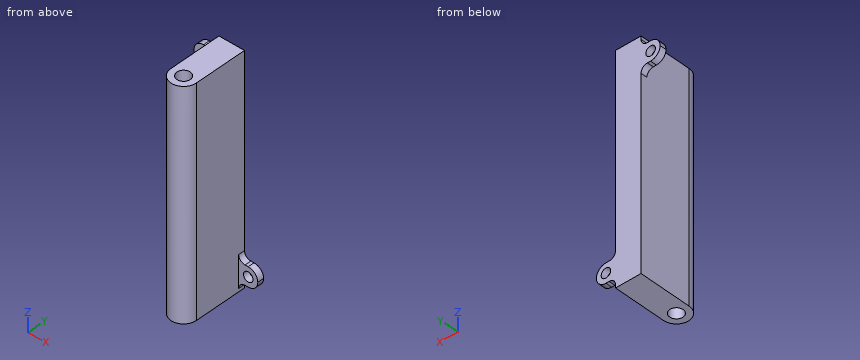
Autodesk Inventor part; units mm, degrees
ref_plane "YZ Plane" through (0, 0, 0) normal (1, 0, 0) x (0, 1, 0)
ref_plane "XZ Plane" through (0, 0, 0) normal (0, 1, 0) x (-1, 0, 0)
ref_plane "XY Plane" through (0, 0, 0) normal (0, 0, 1) x (1, 0, 0)
sketch "Sketch7" plane through (0, 0, 0) normal (0, 0, 1) x (1, 0, 0)
  circle A0 centre (0, 0) radius 4
  arc A1 (-8, 0) -> (8, 0) centre (0, 0) ccw
  line L0 (-8, 29) -> (-20, 29)
  line L1 (-20, 29) -> (-20, 33)
  line L2 (-20, 33) -> (0, 33)
  line L3 (0, 33) -> (20, 33)
  line L4 (20, 33) -> (20, 29)
  line L5 (20, 29) -> (8, 29)
  line L6 (-8, 0) -> (-8, 29)
  line L7 (8, 0) -> (8, 29)
  dimension "d34" = 4
  dimension "d35" = 33
  dimension "d36" = 8
  dimension "d37" = 4
  dimension "d38" = 12
extrude "Extrusion6" add sketch "Sketch7" along normal blind 140
sketch "Sketch8" plane through (-20, 29, 0) normal (0, -1, 0) x (1, 0, 0)
  line L0 (12, 140) -> (0, 140)
  line L1 (0, 0) -> (0, 140)
  line L2 (0, 0) -> (12, 0)
  line L3 (12, 0) -> (12, 140)
  line L4 (40, 140) -> (28, 140)
  line L5 (28, 0) -> (28, 140)
  line L6 (28, 0) -> (40, 0)
  line L7 (40, 0) -> (40, 140)
  line L8 (0, 134) -> (12, 134)
  line L9 (12, 134) -> (12, 122)
  line L10 (12, 122) -> (0, 122)
  line L11 (0, 122) -> (0, 134)
  line L12 (28, 6) -> (40, 6)
  line L13 (40, 6) -> (40, 18)
  line L14 (40, 18) -> (28, 18)
  line L15 (28, 18) -> (28, 6)
  point P0 (20, 0)
  dimension "d41" = 12
  dimension "d42" = 6
  dimension "d43" = 6
extrude "Extrusion7" cut sketch "Sketch8" against normal blind 140 contours L3 L8 L1 L0 | L3 L2 L1 L10 | L7 L14 L5 L4 | L7 L6 L5 L12
fillet "Fillet1" radius 6 4 edges at (20, 31, 6) (20, 31, 18) (-20, 31, 134) (-20, 31, 122)
fillet "Fillet1" radius 4 4 edges at (-8, 31, 134) (-8, 31, 122) (8, 31, 6) (8, 31, 18)
sketch "Sketch9" plane through (-14, 29, 122) normal (0, -1, 0) x (1, 0, 0)
  arc A0 (0, 12) -> (0, 0) centre (0, 6) ccw
  arc A1 (28, -116) -> (28, -104) centre (28, -110) ccw
  line L0 (28, -104) -> (26, -104)
  arc A2 (22, -100) -> (26, -104) centre (26, -100) ccw
  line L1 (22, -120) -> (22, -100)
  arc A3 (26, -116) -> (22, -120) centre (26, -120) ccw
  line L2 (26, -116) -> (28, -116)
  point P0 (14, -122)
hole "Hole2" at (14, 29, 12) at (-14, 29, 128) direction (0, 1, 0) diameter 6 depth 8 tip angle 118
sketch "Sketch10" plane through (0, 0, 140) normal (0, 0, 1) x (1, 0, 0)
  arc A0 (-8, 0) -> (8, 0) centre (0, 0) ccw
hole "Hole3" at (0, 0, 140) direction (0, 0, -1) diameter 8.376 depth 20 tip angle 118
sketch "Sketch11" plane through (0, 0, 0) normal (0, 0, -1) x (-1, 0, 0)
  arc A0 (-8, 0) -> (8, 0) centre (0, 0) ccw
hole "Hole4" at (0, 0, 0) direction (0, 0, 1) diameter 8.376 depth 20 tip angle 118
ref_plane "Work Plane3" through (0, 0, 140) normal (1, 0, 0) x (0, 0, -1)
properties part number "Pusher.Holder" material "Aluminum-6061"
Read the model definition and answer for the solid it produces. Units are mm, in the model's axes. Give positions to 0.01 mm unless a question says otherwise; leave off trailing zeros. Order: outer loops, then holes, each group sorted by start corner. A loop starts at its lowest first (then second) coordinate and runs counter-clockwise, first axis right, second up.
(1) Find section B-B (z = 44). Give the vertices of the cut face in (x, y).
(2) Given pin 1 (5 mm diameter, centred on x = 0, y = 0, fed in from +Z); pin 2 (1 mm diameter, centred on x = -13.5, y = 30, fed in from -Z); pin 3 (9.5 mm diameter, centred on x = 14, z = 12, fed in from -Y); pin 4 (16.5 mm diameter, centred on y = 13.5, z = 69.5, fed in from -X), each flat-ended and moving along its own axis, determine where each tip first touches the part or whether it passes through.
(3) Straight lines are drawn through the part: L1, parallel to Y at x = 0, z = 125; L2, parallel to Z at x = 14, y = 30; L3, parallel to X at y = 0, z = 99. For each, find the intervals that lie inside material, in ascending order.
(4) Find section A-A (x = 0). Give the vertices of the cut face in (y, z).
(5) Find section C-C (y = 7). Give the vertices of the cut face in (x, z).
(6) Find section D-D (x = 6.5). Give the vertices of the cut face in (y, z).
Result sheet:
1. outline: (-8, 0) arc R8 ccw to (8, 0) - (8, 33) - (-8, 33) - close; hole circle Ø8 at (0, 0)
2. pin 1: passes through
2. pin 2: stops at z = 122
2. pin 3: stops at y = 29
2. pin 4: stops at x = -8
3. L1: y = -8 to -4.19, 4.19 to 33
3. L2: z = 6 to 9, 15 to 18
3. L3: x = -8 to -4, 4 to 8
4. outline: (-8, 0) - (-4.19, 0) - (-4.19, 20) - (-4, 20.11) - (-4, 119.89) - (-4.19, 120) - (-4.19, 140) - (-8, 140) - close; (4, 20.11) - (4.19, 20) - (4.19, 0) - (33, 0) - (33, 140) - (4.19, 140) - (4.19, 120) - (4, 119.89) - close
5. outline: (-8, 0) - (8, 0) - (8, 140) - (-8, 140) - close
6. outline: (-4.66, 0) - (33, 0) - (33, 140) - (-4.66, 140) - close
